Verification items for the finished model (mm, model axes). A direction names the side the tool comes from. Give positions to 0.01 mm unless a question says otherwise; leave off trailing zeros. Write each loop counter-clockwise with the first axis right and the second up, starting at its lowest first coordinate (ties: lowest second). Pieces come first, ordered by that corner, then holes. Notation, with made-up numbers: (0, 64.5) -> (54, 64.5) arc R13 ccw to (54, 80.5) -> close; hole circle Ø9 at (-33.75, 0). An arc over 180 degrees is marked (long way). Write item = value, one per line.
from build123d import *

# Parameters (mm, degrees)
SKETCH1_W            = 186.036212306
SKETCH1_H            = 300
BOSS_EXTRUDE1_DEPTH  = 2.5
CUT_EXTRUDE1_DEPTH   = 10
LPATTERN1_COUNT      = 5
LPATTERN1_PITCH      = 25
SKETCH3_W            = 23
SKETCH3_H            = 14.5
CUT_EXTRUDE2_DEPTH   = 10
SKETCH4_R            = 1.5
SKETCH4_W            = 23
SKETCH4_H            = 14.5
CUT_EXTRUDE3_DEPTH   = 10
SKETCH5_W            = 45.5
SKETCH5_H            = 26
CUT_EXTRUDE4_DEPTH   = 10
SKETCH6_W            = 6.5
SKETCH6_H            = 6.5
CUT_EXTRUDE5_DEPTH   = 5
LPATTERN2_COUNT      = 3
LPATTERN2_PITCH      = 25
CUT_EXTRUDE6_DEPTH   = 15
LPATTERN3_COUNT      = 2
LPATTERN3_PITCH      = 20
MIRROR2_COPY_1_DEPTH = 15
CUT_EXTRUDE8_DEPTH   = 15
SKETCH8_W            = 394.980605426
SKETCH8_H            = 443.90792121
SKETCH8_W_2          = 150
SKETCH8_H_2          = 100
CUT_EXTRUDE7_DEPTH   = 15
LPATTERN4_COUNT      = 2
LPATTERN4_PITCH      = 100
SKETCH10_R           = 1.5
CUT_EXTRUDE9_DEPTH   = 15
LPATTERN6_COUNT      = 3
LPATTERN6_PITCH      = 46


with BuildPart() as part:
    # Sketch1 → Boss-Extrude1 (new body)
    with BuildSketch(Plane(origin=(0, 0, 0), x_dir=(1, 0, 0), z_dir=(0, 1, 0))):
        Rectangle(SKETCH1_W, SKETCH1_H)
    extrude(amount=BOSS_EXTRUDE1_DEPTH)

    # Sketch2 → Cut-Extrude1 (cut)
    with BuildSketch(Plane(origin=(0, 2.5, 0), x_dir=(1, 0, 0), z_dir=(0, 1, 0))):
        with BuildLine():
            ThreePointArc((-55.4, -2.376972865), (-50, -5.9), (-44.6, -2.376972865))
            Line((-44.6, -2.376972865), (-44.6, 2.376972865))
            ThreePointArc((-44.6, 2.376972865), (-50, 5.9), (-55.4, 2.376972865))
            Line((-55.4, 2.376972865), (-55.4, -2.376972865))
        make_face()
    cut_extrude1 = extrude(amount=-CUT_EXTRUDE1_DEPTH, mode=Mode.SUBTRACT)

    # LPattern1: Cut-Extrude1 ×5
    with Locations(*[(i * LPATTERN1_PITCH, 0, 0) for i in range(1, LPATTERN1_COUNT)]):
        add(cut_extrude1, mode=Mode.SUBTRACT)

    # Sketch3 → Cut-Extrude2 (cut)
    with BuildSketch(Plane(origin=(0, 2.5, 0), x_dir=(-1, 0, 0), z_dir=(0, 1, 0))):
        with Locations((50, -20)):
            Rectangle(SKETCH3_W, SKETCH3_H)
    cut_extrude2 = extrude(amount=-CUT_EXTRUDE2_DEPTH, mode=Mode.SUBTRACT)

    # Sketch4 → Cut-Extrude3 (cut)
    with BuildSketch(Plane.XZ):
        with Locations(Location((-64, -20, 0), (0, 0, 270))):
            Circle(SKETCH4_R)
        with Locations(Location((-36, -20, 0), (0, 0, 270))):
            Circle(SKETCH4_R)
        with Locations((-50, -20)):
            Rectangle(SKETCH4_W, SKETCH4_H)
    cut_extrude3 = extrude(amount=-CUT_EXTRUDE3_DEPTH, mode=Mode.SUBTRACT)

    # Sketch5 → Cut-Extrude4 (cut)
    with BuildSketch(Plane(origin=(0, 2.5, 0), x_dir=(1, 0, 0), z_dir=(0, 1, 0))):
        with Locations((0, 43)):
            Rectangle(SKETCH5_W, SKETCH5_H)
    extrude(amount=-CUT_EXTRUDE4_DEPTH, mode=Mode.SUBTRACT)

    # Mirror1: Cut-Extrude2, Cut-Extrude3 across plane
    add(cut_extrude2.mirror(Plane(origin=(0, 0, 0), x_dir=(0, 0, 1), z_dir=(1, 0, 0))), mode=Mode.SUBTRACT)
    add(cut_extrude3.mirror(Plane(origin=(0, 0, 0), x_dir=(0, 0, 1), z_dir=(1, 0, 0))), mode=Mode.SUBTRACT)

    # Sketch6 → Cut-Extrude5 (cut)
    with BuildSketch(Plane(origin=(0, 2.5, 0), x_dir=(1, 0, 0), z_dir=(0, 1, 0))):
        with Locations((-25, 12.5)):
            Rectangle(SKETCH6_W, SKETCH6_H)
    cut_extrude5 = extrude(amount=-CUT_EXTRUDE5_DEPTH, mode=Mode.SUBTRACT)

    # LPattern2: Cut-Extrude5 ×3
    with Locations(*[(i * LPATTERN2_PITCH, 0, 0) for i in range(1, LPATTERN2_COUNT)]):
        add(cut_extrude5, mode=Mode.SUBTRACT)

    # Sketch7 → Cut-Extrude6 (cut)
    with BuildSketch(Plane(origin=(0, 2.5, 0), x_dir=(1, 0, 0), z_dir=(0, 1, 0))):
        with BuildLine():
            ThreePointArc((-45.4, 37.623027135), (-40, 34.1), (-34.6, 37.623027135))
            Line((-34.6, 37.623027135), (-34.6, 42.376972865))
            ThreePointArc((-34.6, 42.376972865), (-40, 45.9), (-45.4, 42.376972865))
            Line((-45.4, 42.376972865), (-45.4, 37.623027135))
        make_face()
    cut_extrude6 = extrude(amount=-CUT_EXTRUDE6_DEPTH, mode=Mode.SUBTRACT)

    # LPattern3: Cut-Extrude6 ×2
    with Locations(*[(-i * LPATTERN3_PITCH, 0, 0) for i in range(1, LPATTERN3_COUNT)]):
        add(cut_extrude6, mode=Mode.SUBTRACT)

    # Mirror2: Cut-Extrude6 across plane
    add(cut_extrude6.mirror(Plane(origin=(0, 0, 0), x_dir=(0, 0, 1), z_dir=(1, 0, 0))), mode=Mode.SUBTRACT)

    # Mirror2 copy 1 sketch → Mirror2 copy 1 (cut)
    with BuildSketch(Plane(origin=(20, 2.5, 0), x_dir=(-1, 0, 0), z_dir=(0, 1, 0))):
        with BuildLine():
            ThreePointArc((-45.4, -37.623027135), (-40, -34.1), (-34.6, -37.623027135))
            Line((-34.6, -37.623027135), (-34.6, -42.376972865))
            ThreePointArc((-34.6, -42.376972865), (-40, -45.9), (-45.4, -42.376972865))
            Line((-45.4, -42.376972865), (-45.4, -37.623027135))
        make_face()
    extrude(amount=-MIRROR2_COPY_1_DEPTH, mode=Mode.SUBTRACT)

    # Sketch9 → Cut-Extrude8 (cut)
    with BuildSketch(Plane(origin=(0, 2.5, 0), x_dir=(-1, 0, 0), z_dir=(0, 1, 0))):
        with BuildLine():
            ThreePointArc((47.5, -69.811504727), (50, -70.125), (52.5, -69.811504727))
            Line((52.5, -69.811504727), (52.5, -50.188495273))
            ThreePointArc((52.5, -50.188495273), (50, -49.875), (47.5, -50.188495273))
            Line((47.5, -50.188495273), (47.5, -69.811504727))
        make_face()
        with BuildLine():
            ThreePointArc((47.5, -50.188495273), (50, -49.875), (52.5, -50.188495273))
            Line((52.5, -50.188495273), (52.5, -49.5))
            Line((52.5, -49.5), (47.5, -49.5))
            Line((47.5, -49.5), (47.5, -50.188495273))
        make_face()
        with BuildLine():
            ThreePointArc((47.5, -50.188495273), (39.875, -60), (47.5, -69.811504727))
            Line((47.5, -69.811504727), (47.5, -50.188495273))
        make_face()
        with BuildLine():
            ThreePointArc((52.5, -69.811504727), (57.677657877, -66.600696519), (60.075496266, -61))
            ThreePointArc((60.075496266, -61), (60.112616494, -60.50061228), (60.125, -60))
            ThreePointArc((60.125, -60), (60.112616494, -59.49938772), (60.075496266, -59))
            ThreePointArc((60.075496266, -59), (57.677657877, -53.399303481), (52.5, -50.188495273))
            Line((52.5, -50.188495273), (52.5, -69.811504727))
        make_face()
        with BuildLine():
            Line((60.625, -61), (60.625, -60))
            Line((60.625, -60), (60.625, -59))
            Line((60.625, -59), (60.075496266, -59))
            ThreePointArc((60.075496266, -59), (60.112616494, -59.49938772), (60.125, -60))
            ThreePointArc((60.125, -60), (60.112616494, -60.50061228), (60.075496266, -61))
            Line((60.075496266, -61), (60.625, -61))
        make_face()
        with BuildLine():
            Line((52.5, -70.5), (52.5, -69.811504727))
            ThreePointArc((52.5, -69.811504727), (50, -70.125), (47.5, -69.811504727))
            Line((47.5, -69.811504727), (47.5, -70.5))
            Line((47.5, -70.5), (52.5, -70.5))
        make_face()
    cut_extrude8 = extrude(amount=-CUT_EXTRUDE8_DEPTH, mode=Mode.SUBTRACT)

    # Sketch8 → Cut-Extrude7 (cut)
    with BuildSketch(Plane(origin=(0, 2.5, 0), x_dir=(1, 0, 0), z_dir=(0, 1, 0))):
        with Locations((0, 32.5)):
            Rectangle(SKETCH8_W, SKETCH8_H)
        with Locations((0, 32.5)):
            Rectangle(SKETCH8_W_2, SKETCH8_H_2, mode=Mode.SUBTRACT)
    extrude(amount=-CUT_EXTRUDE7_DEPTH, mode=Mode.SUBTRACT)

    # LPattern4: Cut-Extrude8 ×2
    with Locations(*[(i * LPATTERN4_PITCH, 0, 0) for i in range(1, LPATTERN4_COUNT)]):
        add(cut_extrude8, mode=Mode.SUBTRACT)

    # Sketch10 → Cut-Extrude9 (cut)
    with BuildSketch(Plane(origin=(0, 2.5, 0), x_dir=(1, 0, 0), z_dir=(0, 1, 0))):
        with Locations(Location((-71, 78.5, 0), (0, 0, 270))):
            Circle(SKETCH10_R)
        with Locations(Location((71, 78.5, 0), (0, 0, 270))):
            Circle(SKETCH10_R)
        with Locations(Location((0, 78.5, 0), (0, 0, 270))):
            Circle(SKETCH10_R)
    cut_extrude9 = extrude(amount=-CUT_EXTRUDE9_DEPTH, mode=Mode.SUBTRACT)

    # LPattern6: Cut-Extrude9 ×3
    with Locations(*[(0, 0, i * LPATTERN6_PITCH) for i in range(1, LPATTERN6_COUNT)]):
        add(cut_extrude9, mode=Mode.SUBTRACT)


solid = part.part
Item 1: Sectioned sample at A-A on x = 0. Record the cut outline in (y, z).
Response values:
outline = (0, -82.5) -> (2.5, -82.5) -> (2.5, -80) -> (0, -80) -> close; (0, -77) -> (2.5, -77) -> (2.5, -56) -> (0, -56) -> close; (0, -30) -> (2.5, -30) -> (2.5, -15.75) -> (0, -15.75) -> close; (0, -9.25) -> (2.5, -9.25) -> (2.5, -5.9) -> (0, -5.9) -> close; (0, 5.9) -> (2.5, 5.9) -> (2.5, 12) -> (0, 12) -> close; (0, 15) -> (2.5, 15) -> (2.5, 17.5) -> (0, 17.5) -> close
Item 2: Set-up check for faces 3 (the cylindrical face through (59.9, 1.3, -45.9)), 4 (the flat face through (-1, 2.5, -22)): record each of +Z, -Z, +X, -X, +Y, -Y from which the full face is reachable in a straight line by a thin tool's end or side.
Response values:
face_3 = +Y, -Y
face_4 = +Z, -Z, +X, -X, +Y
Item 3: Material ranges on line 1 (X direction, y = 1.7, z = 13.5); line 2 (Z direction, x = -71, y = 1.5); line 3 (X direction, y = 0.9, z = -32.5), recorded low to high.
Response values:
line_1 = -75 to -72.5, -69.5 to -1.5, 1.5 to 69.5, 72.5 to 75
line_2 = -82.5 to -80, -77 to -34, -31 to 12, 15 to 17.5
line_3 = -75 to -72.5, -69.5 to -22.75, 22.75 to 69.5, 72.5 to 75
Item 4: Sectioned sample at B-B on z = -32.5. Record the cut outline in (x, y).
Response values:
outline = (-75, 0) -> (-72.5, 0) -> (-72.5, 2.5) -> (-75, 2.5) -> close; (-69.5, 0) -> (-22.75, 0) -> (-22.75, 2.5) -> (-69.5, 2.5) -> close; (22.75, 0) -> (69.5, 0) -> (69.5, 2.5) -> (22.75, 2.5) -> close; (72.5, 0) -> (75, 0) -> (75, 2.5) -> (72.5, 2.5) -> close
Item 5: Go/stop test with flat-tipped pins: P1, Ø3.5, axis at x = 0, z = -78.5, coming from the +Y side; P2, Ø2.5, axis at x = 36, z = -20, coming from the -Y side. Record where each tip stops, or that it passes through.
Response values:
P1 = 2.5
P2 = through
Item 6: Mould release check, pull along Z, two halves, no side actions. Record for faces 1 (the cylindrical face through (-57.62, 1.27, -66.67)), 2 (the flat face through (-1, 0, -22)): +Z half, -Z half, draft (parallel to the pull), parting line (faces both ways), or undercut.
Response values:
face_1 = undercut
face_2 = draft
Item 7: Sectioned sample at D-D on x = -51. Record the cut outline in (y, z).
Response values:
outline = (0, -82.5) -> (2.5, -82.5) -> (2.5, -70.5) -> (0, -70.5) -> close; (0, -49.5) -> (2.5, -49.5) -> (2.5, -27.25) -> (0, -27.25) -> close; (0, -12.75) -> (2.5, -12.75) -> (2.5, -5.81) -> (0, -5.81) -> close; (0, 5.81) -> (2.5, 5.81) -> (2.5, 17.5) -> (0, 17.5) -> close
Item 8: Sectioned sample at C-C on z = -63. Record the cut outline in (x, y).
Response values:
outline = (-75, 0) -> (-59.67, 0) -> (-59.67, 2.5) -> (-75, 2.5) -> close; (-40.33, 0) -> (40.33, 0) -> (40.33, 2.5) -> (-40.33, 2.5) -> close; (59.67, 0) -> (75, 0) -> (75, 2.5) -> (59.67, 2.5) -> close
